Design review of the part built by this model. Coordinates are the model's own, in mm. A direction names the side the tool comes from. Round coordinates to 2 decimals unless told otherwise and drop trailing zeros. Loops run counter-clockwise (first coordinate to the right, second up) from the corner with the lowest first, then second, coordinate; pieces in that order, holes last. Notation, with made-up numbers: (6.5, -22) -> (62.5, -22) arc R21 ccw to (62.5, -8) -> close; hole circle Ø5 at (-19.75, -34.5). An arc over 180 degrees is marked (long way). Use a Markdown table: item, result. Add a question column.
Autodesk Inventor part; units mm, degrees
ref_plane "YZ Plane" through (0, 0, 0) normal (1, 0, 0) x (0, 1, 0)
ref_plane "XZ Plane" through (0, 0, 0) normal (0, 1, 0) x (-1, 0, 0)
ref_plane "XY Plane" through (0, 0, 0) normal (0, 0, 1) x (1, 0, 0)
sketch "Эскиз5" plane through (0, 0, 0) normal (0, 0, 1) x (1, 0, 0)
  line L0 (0, 0) -> (-20, 0)
  line L1 (-20, 0) -> (-20, 25)
  line L2 (-16, 29) -> (-4, 29)
  line L3 (0, 25) -> (0, 0)
  line L4 (-4, 29) -> (0, 25)
  line L5 (-16, 29) -> (-20, 25)
  point P0 (-20, 29)
  point P1 (0, 29)
  dimension "d35" = 20
  dimension "d36" = 29
  dimension "d37" = 4
  dimension "d38" = 4
  dimension "d39" = 4
  dimension "d40" = 4
revolve "Вращение3" add sketch "Эскиз5" angle 360 about axis through (0, 0, 0) along (-1, 0, 0)
sketch "Эскиз6" plane through (0, 0, 0) normal (1, 0, 0) x (0, 0, -1)
  line L0 (0, 0) -> (0, 23) construction
  dimension "d42" = 23
hole "Отверстие2" at (0, 23, 0) direction (-1, 0, 0) diameter 4 depth 4
sketch "Эскиз7" plane through (0, 0, 0) normal (1, 0, 0) x (0, 0, -1)
  point P0 (0, 0)
  point P1 (0, 0)
hole "Отверстие3" at (0, 0, 0) direction (-1, 0, 0) diameter 16 depth 8 tip angle 140 countersink diameter 18 countersink angle 90
sketch "Эскиз8" plane through (0, 0, 0) normal (0, 0, 1) x (1, 0, 0)
  line L0 (-20, -25) -> (-20, 25) construction
  line L1 (-20, 2) -> (-14, 2)
  line L2 (-14, 2) -> (-14, -2)
  line L3 (-14, -2) -> (-20, -2)
  line L4 (-20, -2) -> (-20, 2)
  point P0 (0, 0)
  point P1 (-20, 0)
  point P2 (-20, 0)
  dimension "d57" = 6
  dimension "d58" = 4
extrude "Выдавливание2" cut sketch "Эскиз8" along normal through all both and the other way through all
thread "Резьба3"
properties part number "711137"
1. Consider section A-A on x = -2.75. State the section outline as (y, z) points, plus the area to 3 significant figures.
2. Mouldability with a two-part tool opening along Y and no side actions: class faces 1 (the face through (-19.75, -25.245, 0.531)), 2 (the face through (-9.92, 13.38, -25.73)), 3 (the face through (-4, 23, 0)) as +Y half, -Y half, draft (parallel to the pull), parting line (faces both ways), or undercut.
3. Insertion check: P1, Ø8, axis at x = -11.5, z = -13, coming from the +Y side; P2, Ø1.5, axis at x = -3.5, y = -16.5, coming from the +Z side; P3, Ø1, axis at x = -6, y = -14, coming from the -Z side. Each pin has a flat end and moves straight along its axis. Give the tip position at first contact, or say it passes through.
4. For faces 4 (the face through (-4.55, 7.81, 1.73)), 5 (the face through (-20, 11, 0)), 6 (the face through (-17, -2, 0)), list the 3-axis set-ups (+Z, -Z, +X, -X, +Y, -Y) from which the entire face can be reached by the end or side of a thin tool; tool diameter is ignored.
5. To check wall thickness, follow probe 1 along Y at (x, z) = (-1.8, 0); probe 2 along Z at (x, y) = (-5.25, 0); probe 3 along Y at (x, z) = (-3.15, 0). State the ranges of each line that lie inside material, in increasing order. Write a range as from..to.
6. Consider section B-B on x = -13.25. State the section outline as (y, z) points.
Verdict:
| question | item | result |
|---|---|---|
| 1 | outline | circle Ø55.5 at (0, 0); hole circle Ø16 at (0, 0); hole circle Ø4 at (23, 0) |
| 1 | area | 2,210 mm² |
| 2 | face 1 | -Y half |
| 2 | face 2 | parting line |
| 2 | face 3 | undercut |
| 3 | P1 | stops at y = 27.57 |
| 3 | P2 | stops at z = 24.23 |
| 3 | P3 | stops at z = -25.67 |
| 4 | face 4 | +X |
| 4 | face 5 | +Z, -Z, -X, +Y, -Y |
| 4 | face 6 | +Z, -Z, -X |
| 5 | probe 1 | y = -26.8..-8, 8..21, 25..26.8 |
| 5 | probe 2 | z = -29..-8, 8..29 |
| 5 | probe 3 | y = -28.15..-8, 8..21, 25..28.15 |
| 6 | outline | circle Ø58 at (0, 0) |
